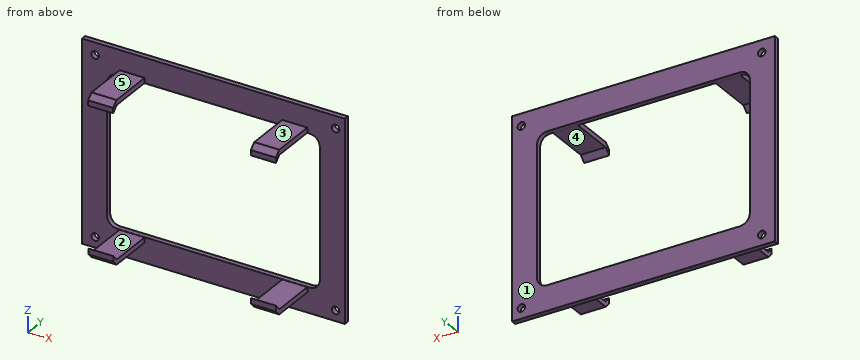
```python
from build123d import *

# Parameters (mm, degrees)
F0_W      = 105
F0_H      = 80
F0_W_2    = 10
F0_H_2    = 2
F1_DEPTH  = 2
F2_D      = 3
F3_DEPTH  = 20
F5_DEPTH  = 10
F7_DEPTH  = 10
F9_DEPTH  = 10
F11_DEPTH = 10


with BuildPart() as f1:
    # F0 (on Front) → F1 (new body)
    with BuildSketch(Plane.XZ):
        with Locations((4.4443034394, -0.1203698614)):
            Rectangle(F0_W, F0_H)
        with Locations((-28.0556965606, -31.2203698614)):
            Rectangle(F0_W_2, F0_H_2, mode=Mode.SUBTRACT)
        with Locations((36.9443034394, -31.2203698614)):
            Rectangle(F0_W_2, F0_H_2, mode=Mode.SUBTRACT)
        with Locations((-28.0556965606, 30.9796301386)):
            Rectangle(F0_W_2, F0_H_2, mode=Mode.SUBTRACT)
        with BuildLine():
            ThreePointArc((-38.0556965606, 25.8796301386), (-36.8841236853, 28.7080572633), (-34.0556965606, 29.8796301386))
            Line((-34.0556965606, 29.8796301386), (42.9443034394, 29.8796301386))
            ThreePointArc((42.9443034394, 29.8796301386), (45.7727305642, 28.7080572633), (46.9443034394, 25.8796301386))
            Line((46.9443034394, 25.8796301386), (46.9443034394, -26.1203698614))
            ThreePointArc((46.9443034394, -26.1203698614), (45.7727305642, -28.9487969862), (42.9443034394, -30.1203698614))
            Line((42.9443034394, -30.1203698614), (-34.0556965606, -30.1203698614))
            ThreePointArc((-34.0556965606, -30.1203698614), (-36.8841236853, -28.9487969862), (-38.0556965606, -26.1203698614))
            Line((-38.0556965606, -26.1203698614), (-38.0556965606, 25.8796301386))
        make_face(mode=Mode.SUBTRACT)
        with Locations((36.9443034394, 30.9796301386)):
            Rectangle(F0_W_2, F0_H_2, mode=Mode.SUBTRACT)
    extrude(amount=F1_DEPTH)

    # F2 (through all)
    with Locations(Plane(origin=(0, 0, 0), x_dir=(1, 0, 0), z_dir=(0, 1, 0))):
        with Locations((-42.8249463439, -34.9864512682), (-42.8249463439, 35.9423682094), (53.229637444, 35.9423682094), (53.229637444, -34.9864512682)):
            Hole(F2_D / 2)

    # F0 (on Front) → F3 (join)
    with BuildSketch(Plane.XZ):
        with Locations((-28.0556965606, 30.9796301386)):
            Rectangle(F0_W_2, F0_H_2)
        with Locations((36.9443034394, 30.9796301386)):
            Rectangle(F0_W_2, F0_H_2)
        with Locations((-28.0556965606, -31.2203698614)):
            Rectangle(F0_W_2, F0_H_2)
        with Locations((36.9443034394, -31.2203698614)):
            Rectangle(F0_W_2, F0_H_2)
    extrude(amount=F3_DEPTH)

    # F4 (on face) → F5 (join)
    with BuildSketch(Plane(origin=(-33.0556965606, 0, 0), x_dir=(0, -1, 0), z_dir=(-1, 0, 0))):
        Polygon((20, 31.9796301386), (20, 29.9796301386), (22.2622127322, 27.8908082008), (22.2622127322, 29.9796301386), align=None)
    extrude(amount=-F5_DEPTH)

    # F6 (on face) → F7 (join)
    with BuildSketch(Plane(origin=(-33.0556965606, 0, 0), x_dir=(0, -1, 0), z_dir=(-1, 0, 0))):
        Polygon((22.0167362937, -27.9179245889), (20, -30.2203698614), (20, -32.2203698614), (22.0167362937, -30.2203698614), align=None)
    extrude(amount=-F7_DEPTH)

    # F8 (on face) → F9 (join)
    with BuildSketch(Plane.YZ.offset(41.9443034394)):
        Polygon((-22.2486329954, 27.8861031592), (-20, 29.9796301386), (-20, 31.9796301386), (-22.2486329954, 29.9796301386), align=None)
    extrude(amount=-F9_DEPTH)

    # F10 (on face) → F11 (join)
    with BuildSketch(Plane.YZ.offset(41.9443034394)):
        Polygon((-21.9842810184, -30.2190438569), (-20, -32.2203698614), (-20, -30.2203698614), (-21.9842810184, -27.9021759242), align=None)
    extrude(amount=-F11_DEPTH)


solid = f1.part
```
The model under review builds one solid part; all positions refer to its coordinate system, in mm. Face numbers are marked on the shaded views. A direction names the side the tool comes from. Give positions to 0.01 mm unless a question says otherwise; leave off trailing zeros. Write each loop counter-clockwise with the first axis right and the second up, starting at its lowest first coordinate (ties: lowest second). Pieces come first, ordered by that corner, then holes. Notation, with made-up numbers: M 62,-28 L 105,-28 A21 ccw 105,-22 Z; hole C -31,-23.5 d1. An arc over 180 degrees is marked long. Write item = value, one per line. Start each with the question number.
Q1. Clearance check with flat-ended pins moving along their axes: pin 1 (10 mm diameter, centred on y = -13.5, z = -30, fed in from +X); pin 2 (1.3 mm diameter, centred on y = -13.5, z = -30.5, fed in from -X); pin 3 (11 mm diameter, centred on x = 35.5, y = -13.5, fed in from -Z); pin 4 (10 mm diameter, centred on x = 15, y = -10, fed in from +Z). State where each tip first meets the part, or that it passes through.
Q2. For line 1 (X direction, y = -19, z = -31.5); line 2 (Z direction, x = 32.5, y = -9.25); line 3 (Y direction, x = -43, z = 10.5), list the stretches that pass through material, from the lowest coordinate up.
Q3. We need section D-D (x = 48.5). State the section outline as (y, z) points.
Q4. We need section A-A (z = 23). State the section outline as (x, y) points, plus the area to 3 significant figures.
Q5. We need section C-C (x = 13.5). State the section outline as (y, z) points.
Q6. Machinability: for the marked faces 4 and 5, which of the approach directions +Z, -Z, +X, -X, +Y, -Y give a long, thin tool a straight path to every point of the face, cutting with its end or side? Answer none if there is none.
Q7. Mouldability with a two-part tool opening along Y and no side actions: class the marked faces 1, 2 and 3 as released by +Y, released by -Y, zero draft, split by the parting line, or undercut.
Q8. We need section B-B (y = -3.75). State the section outline as (x, z) points, plus the area to 3 significant figures.
Result set:
q1.pin_1 = 41.94
q1.pin_2 = -33.06
q1.pin_3 = -32.22
q1.pin_4 = through
q2.line_1 = -33.06 to -23.06, 31.94 to 41.94
q2.line_2 = -32.22 to -30.22, 29.98 to 31.98
q2.line_3 = -2 to 0
q3.outline = M -2,-40.12 L 0,-40.12 L 0,39.88 L -2,39.88 Z
q4.outline = M -48.06,-2 L -38.06,-2 L -38.06,0 L -48.06,0 Z; M 46.94,-2 L 56.94,-2 L 56.94,0 L 46.94,0 Z
q4.area = 40.0 mm2
q5.outline = M -2,-40.12 L 0,-40.12 L 0,-30.12 L -2,-30.12 Z; M -2,29.88 L 0,29.88 L 0,39.88 L -2,39.88 Z
q6.face_4 = +X, -X
q6.face_5 = +Z, +X, -X, -Y
q7.face_1 = released by +Y
q7.face_2 = undercut
q7.face_3 = zero draft
q8.outline = M -33.06,-32.22 L -23.06,-32.22 L -23.06,-30.22 L -33.06,-30.22 Z; M -33.06,29.98 L -23.06,29.98 L -23.06,31.98 L -33.06,31.98 Z; M 31.94,-32.22 L 41.94,-32.22 L 41.94,-30.22 L 31.94,-30.22 Z; M 31.94,29.98 L 41.94,29.98 L 41.94,31.98 L 31.94,31.98 Z
q8.area = 80.0 mm2
